```python
from build123d import *

# Parameters (mm, degrees)
SKETCH_1_W           = 99.974800609
SKETCH_1_H           = 51.97470409
EXTRUDE_1_DEPTH      = 8.6
SKETCH_2_W           = 95.974800609
SKETCH_2_H           = 47.97470409
CUT_EXTRUDE_1_DEPTH  = 4
SKETCH_3_W           = 2
SKETCH_3_H           = 10
SKETCH_3_H_2         = 9.97470409
CUT_EXTRUDE_2_DEPTH  = 3.35
SKETCH_4_R           = 1.1
SKETCH_4_W           = 38.392586289
SKETCH_4_H           = 7.4
SKETCH_4_W_2         = 5.95
SKETCH_4_H_2         = 5.95
CUT_EXTRUDE_3_DEPTH  = 1437.448457956
FILLET_1_R           = 3
FILLET_3_R           = 2
SKETCH_7_W           = 53.6
SKETCH_7_H           = 10.97470409
CUT_EXTRUDE_14_DEPTH = 4
FILLET_7_R           = 2
FILLET_8_R           = 1
SKETCH_14_W          = 2.323736835
SKETCH_14_H          = 6.8
CUT_EXTRUDE_15_DEPTH = 2
SKETCH_15_W          = 4.3
SKETCH_15_H          = 51.97470409
CUT_EXTRUDE_16_DEPTH = 1490.156636733
SKETCH_6_W           = 6.76
SKETCH_6_H           = 6.795709929
CUT_EXTRUDE_17_DEPTH = 4


with BuildPart() as part:
    # 草图1 → 凸台-拉伸1 (new body)
    with BuildSketch(Plane.XY.offset(1046.483288979)):
        with Locations((934.375963031, 1020.144466268)):
            Rectangle(SKETCH_1_W, SKETCH_1_H)
    extrude(amount=EXTRUDE_1_DEPTH)

    # 草图2 → 切除-拉伸1 (cut)
    with BuildSketch(Plane(origin=(0, 0, 1046.483288979), x_dir=(-1, 0, 0), z_dir=(0, 0, -1))):
        with Locations((-934.375963031, 1020.144466268)):
            Rectangle(SKETCH_2_W, SKETCH_2_H)
    extrude(amount=-CUT_EXTRUDE_1_DEPTH, mode=Mode.SUBTRACT)

    # 草图3 → 切除-拉伸2 (cut)
    with BuildSketch(Plane(origin=(0, 0, 1046.483288979), x_dir=(-1, 0, 0), z_dir=(0, 0, -1))):
        with Locations((-885.388562726, 1034.131818313)):
            Rectangle(SKETCH_3_W, SKETCH_3_H)
        with Locations((-885.388562726, 1020.144466268)):
            Rectangle(SKETCH_3_W, SKETCH_3_H_2)
        with Locations((-885.388562726, 1006.157114223)):
            Rectangle(SKETCH_3_W, SKETCH_3_H)
    extrude(amount=-CUT_EXTRUDE_2_DEPTH, mode=Mode.SUBTRACT)

    # 草图4 → 切除-拉伸3 (cut, through all)
    with BuildSketch(Plane(origin=(0, 0, 1050.483288979), x_dir=(-1, 0, 0), z_dir=(0, 0, -1))):
        with Locations((-920.388562726, 1041.631818313)):
            Circle(SKETCH_4_R)
        with Locations((-920.388562726, 998.657114223)):
            Circle(SKETCH_4_R)
        with Locations((-972.363363335, 998.657114223)):
            Circle(SKETCH_4_R)
        with Locations((-972.363363335, 1041.631818313)):
            Circle(SKETCH_4_R)
        with Locations((-949.933821712, 1001.144429438)):
            Rectangle(SKETCH_4_W, SKETCH_4_H)
        with Locations((-977.376048121, 1035.144495478)):
            Rectangle(SKETCH_4_W_2, SKETCH_4_H_2)
    extrude(amount=-CUT_EXTRUDE_3_DEPTH, mode=Mode.SUBTRACT)

    # 圆角1
    fillet_1_edges = [part.edges().sort_by_distance(p)[0] for p in [
        (884.388562726, 1046.131818313, 1050.783288979),
        (984.363363335, 1046.131818313, 1050.783288979),
        (984.363363335, 994.157114223, 1050.783288979),
        (884.388562726, 994.157114223, 1050.783288979),
    ]]
    fillet(fillet_1_edges, radius=FILLET_1_R)

    # 圆角3
    fillet_3_edges = [part.edges().sort_by_distance(p)[0] for p in [
        (980.351048121, 1032.169495478, 1052.783288979),
        (980.351048121, 1038.119495478, 1052.783288979),
        (974.401048121, 1038.119495478, 1052.783288979),
        (974.401048121, 1032.169495478, 1052.783288979),
    ]]
    fillet(fillet_3_edges, radius=FILLET_3_R)

    # 草图7 → 切除-拉伸14 (cut)
    with BuildSketch(Plane.XY.offset(1055.083288979)):
        Polygon((885.888562726, 1019.831818313), (982.863363335, 1019.831818313), (982.863363335, 1008.131818313), (927.763363335, 1008.131818313), (927.763363335, 1006.631818313), (927.763363335, 995.657114223), (885.888562726, 995.657114223), align=None)
        Polygon((934.163363335, 1044.631818313), (934.163363335, 1033.131818313), (935.663363335, 1033.131818313), (935.663363335, 1044.631818313), (982.863363335, 1044.631818313), (982.863363335, 1021.331818313), (963.463363335, 1021.331818313), (963.463363335, 1032.731818313), (943.963363335, 1032.731818313), (943.963363335, 1031.231818313), (961.963363335, 1031.231818313), (961.963363335, 1021.331818313), (927.563363335, 1021.331818313), (927.563363335, 1032.811818313), (904.363363335, 1032.811818313), (904.363363335, 1044.631818313), align=None)
        with Locations((956.063363335, 1001.144466268)):
            Rectangle(SKETCH_7_W, SKETCH_7_H)
        Polygon((926.063363335, 1021.331818313), (926.063363335, 1031.311818313), (902.863363335, 1031.311818313), (902.863363335, 1044.631818313), (885.888562726, 1044.631818313), (885.888562726, 1021.331818313), align=None)
    extrude(amount=-CUT_EXTRUDE_14_DEPTH, mode=Mode.SUBTRACT)

    # 圆角7
    fillet_7_edges = [part.edges().sort_by_distance(p)[0] for p in [
        (982.363363335, 996.157114223, 1048.483288979),
        (982.363363335, 1044.131818313, 1048.483288979),
        (886.388562726, 1044.131818313, 1048.483288979),
        (886.388562726, 996.157114223, 1048.483288979),
        (982.863363335, 995.657114223, 1053.083288979),
        (929.263363335, 995.657114223, 1053.083288979),
        (929.263363335, 1006.631818313, 1053.083288979),
        (982.863363335, 1006.631818313, 1053.083288979),
        (961.963363335, 1021.331818313, 1053.083288979),
        (927.563363335, 1021.331818313, 1053.083288979),
        (927.563363335, 1032.811818313, 1053.083288979),
        (904.363363335, 1032.811818313, 1053.083288979),
        (904.363363335, 1044.631818313, 1053.083288979),
        (934.163363335, 1044.631818313, 1053.083288979),
        (935.663363335, 1044.631818313, 1053.083288979),
        (982.863363335, 1044.631818313, 1053.083288979),
        (982.863363335, 1021.331818313, 1053.083288979),
        (963.463363335, 1021.331818313, 1053.083288979),
        (963.463363335, 1032.731818313, 1053.083288979),
        (961.963363335, 1031.231818313, 1053.083288979),
        (885.888562726, 1021.331818313, 1053.083288979),
        (885.888562726, 1044.631818313, 1053.083288979),
        (902.863363335, 1044.631818313, 1053.083288979),
        (902.863363335, 1031.311818313, 1053.083288979),
        (926.063363335, 1031.311818313, 1053.083288979),
        (926.063363335, 1021.331818313, 1053.083288979),
        (927.763363335, 995.657114223, 1053.083288979),
        (885.888562726, 995.657114223, 1053.083288979),
        (885.888562726, 1019.831818313, 1053.083288979),
        (982.863363335, 1019.831818313, 1053.083288979),
        (982.863363335, 1008.131818313, 1053.083288979),
        (927.763363335, 1008.131818313, 1053.083288979),
    ]]
    fillet(fillet_7_edges, radius=FILLET_7_R)

    # 圆角8
    fillet_8_edges = [part.edges().sort_by_distance(p)[0] for p in [
        (930.737528567, 997.444429438, 1050.783288979),
        (969.130114856, 997.444429438, 1050.783288979),
        (930.737528567, 1004.844429438, 1050.783288979),
        (969.130114856, 1004.844429438, 1050.783288979),
    ]]
    fillet(fillet_8_edges, radius=FILLET_8_R)

    # 草图14 → 切除-拉伸15 (cut)
    with BuildSketch(Plane.XY.offset(1055.083288979)):
        with Locations((983.201494917, 1013.231818313)):
            Rectangle(SKETCH_14_W, SKETCH_14_H)
    extrude(amount=-CUT_EXTRUDE_15_DEPTH, mode=Mode.SUBTRACT)

    # 草图15 → 切除-拉伸16 (cut, through all)
    with BuildSketch(Plane(origin=(984.363363335, 0, 0), x_dir=(0, 0, -1), z_dir=(1, 0, 0))):
        with Locations((-1052.933288979, 1020.144466268)):
            Rectangle(SKETCH_15_W, SKETCH_15_H)
    extrude(amount=-CUT_EXTRUDE_16_DEPTH, mode=Mode.SUBTRACT)

    # 草图6 → 切除-拉伸17 (cut)
    with BuildSketch(Plane(origin=(0, 0, 1046.483288979), x_dir=(-1, 0, 0), z_dir=(0, 0, -1))):
        with Locations((-926.946347841, 997.554969188)):
            Rectangle(SKETCH_6_W, SKETCH_6_H)
    extrude(amount=-CUT_EXTRUDE_17_DEPTH, mode=Mode.SUBTRACT)


solid = part.part
```
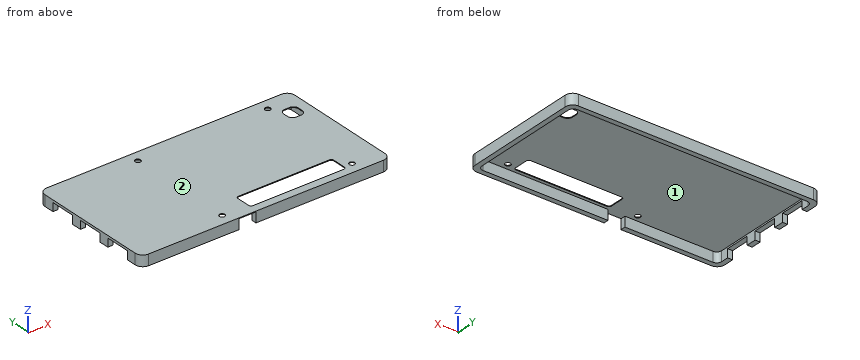
Build history of the part. All positions in model axes, mm. Face numbers are marked on the shaded views. Coordinates: 2 decimals unless noted, no trailing zeros. Order: outer loops, then holes, each group sorted by start corner. A loop starts at its lowest first (then second) coordinate and runs counter-clockwise, first axis right, second up.
Item 1: Saw through at A-A on x = 967. List the corners of the cut face in (y, z), then the cut area to 3 significant figures.
Filled in:
outline: (994.16, 1046.48) - (996.16, 1046.48) - (996.16, 1050.48) - (997.44, 1050.48) - (997.44, 1050.78) - (994.16, 1050.78) - close; (1004.84, 1050.48) - (1044.13, 1050.48) - (1044.13, 1046.48) - (1046.13, 1046.48) - (1046.13, 1050.78) - (1004.84, 1050.78) - close
area: 29.4 mm2
Item 2: Drill centre lines: L1, parallel to Y at x = 917, z = 1049.35; L2, parallel to X at y = 1026.5, z = 1049; L3, parallel to X at y = 1034, z = 1050.6. Where is each one in solid material? Low to high.
Filled in:
L1: y = 994.16 to 996.16, 1044.13 to 1046.13
L2: x = 884.39 to 886.39, 982.36 to 984.36
L3: x = 884.39 to 974.41, 980.34 to 984.36
Item 3: Saw through at B-B on y = 1026.5. List the corners of the cut face in (x, z), then the cut area to 3 significant figures.
Filled in:
outline: (884.39, 1046.48) - (886.39, 1046.48) - (886.39, 1050.48) - (982.36, 1050.48) - (982.36, 1046.48) - (984.36, 1046.48) - (984.36, 1050.78) - (884.39, 1050.78) - close
area: 46.0 mm2
Item 4: Saw through at C-C on z = 1048. State how many separate pieces and enclosed holes the cut face has, then the cut area to 3 significant figures.
Filled in:
separate pieces: 4
enclosed holes: 0
area: 514 mm2
Item 5: Mould opens along Y. For the marked faces 1 and 2 say: released by +Y, released by -Y, zero draft, split by the parting line, or undercut.
Filled in:
face 1: undercut
face 2: zero draft
Item 6: Saw through at D-D on x = 911. List the corners of the cut face in (y, z).
Filled in:
outline: (994.16, 1046.48) - (996.16, 1046.48) - (996.16, 1050.48) - (1044.13, 1050.48) - (1044.13, 1046.48) - (1046.13, 1046.48) - (1046.13, 1050.78) - (994.16, 1050.78) - close
Item 7: Drop flat-ended pins along their axis: pin 1 Ø1.6 at (x, y) = (885.5, 1004) entering from -Z; pin 2 Ø0.6 at (y, z) = (995, 1048.5) entering from -X; pin 3 Ø1 at (x, z) = (885.5, 1047.5) entering from +Y. Give the stop position or say it passes through.
Filled in:
pin 1: stops at z = 1049.83
pin 2: stops at x = 885.03
pin 3: stops at y = 1045.79
